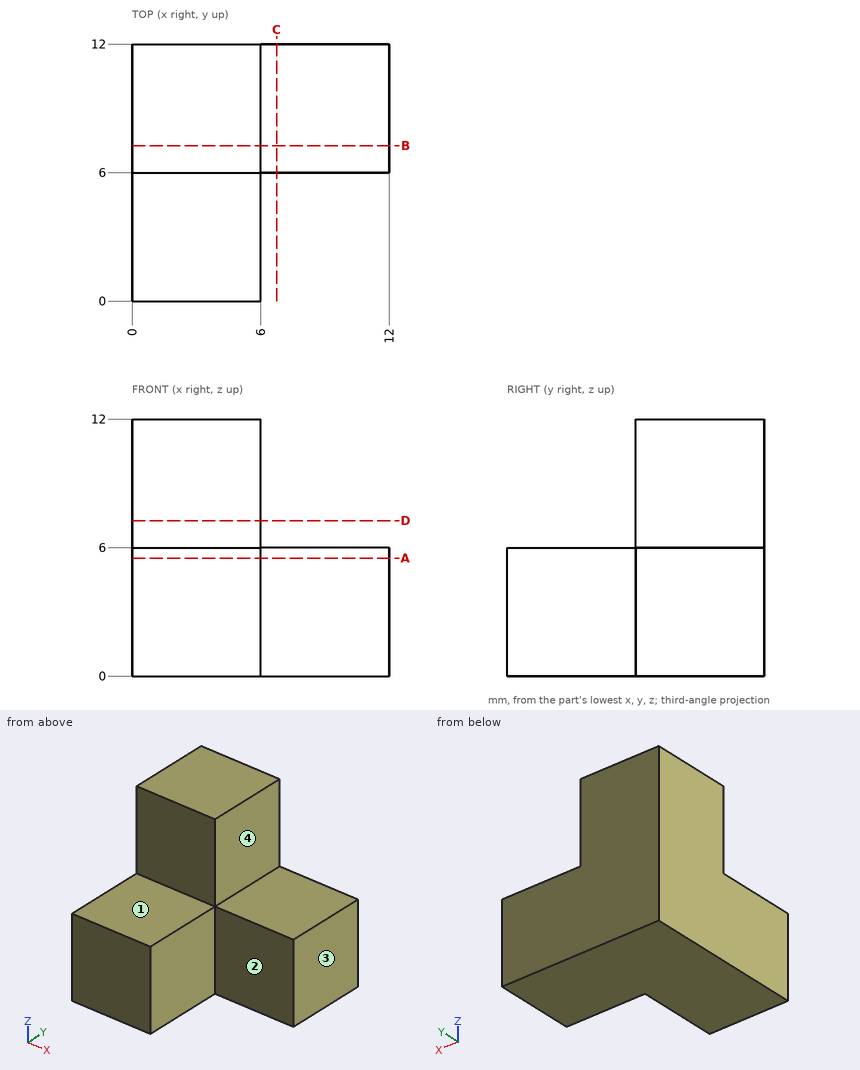
Study the drawing (mm; zero at the part's minimum x, y, z) and answer. A direction names the side the tool comes from. Coordinates: 2 decimals unless noted, no trailing zeros. Write each loop counter-clockwise with the first axis right and the second up, starting at its lowest first coordinate (ties: lowest second). Pieces come first, ordered by that corner, then holes. Notation, with made-up numbers: M -24.75,53 L 33.25,53 A36 ccw 33.25,89 Z; hole C 44.25,43 d10. An arc over 180 degrees is marked long. Use a Markdown table: item, result. Add a question column.
1. Section C-C (x = 6.75) is taken. Give the vertices of the cut face in (y, z), plus the area to 3 significant figures.
2. Section B-B (y = 7.25) is taken. Give the vertices of the cut face in (x, z), plus the area to 3 significant figures.
3. Section D-D (z = 7.25) is taken. Give the vertices of the cut face in (x, y).
4. Given P1, Ø3, axis at y = 4, z = 2, coming from the +X side; P2, Ø1.8, axis at x = 9.5, z = 3.5, coming from the -Y side; P3, Ø3, axis at x = 2.5, y = 3.5, coming from the +Z side, each flat-ended and moving along its own axis, determine where each tip first touches the part or whether it passes through.
5. Straight lines are drawn through the part: line 1 along Y through (x, z) = (2, 11); line 2 along X through (y, z) = (8.75, 11). For each, find the intervals that lie inside material, in ascending order. Write a range as [from, to].
6. Section A-A (z = 5.5) is taken. Give the vertices of the cut face in (x, y).
7. Which of the six approach directions +Z, -Z, +X, -X, +Y, -Y give full straight-line access (tool end or side, diameter ignored) to the marked faces 1, 2, 3 and 4?
Data:
| question | item | result |
|---|---|---|
| 1 | outline | M 6,0 L 12,0 L 12,6 L 6,6 Z |
| 1 | area | 36.0 mm2 |
| 2 | outline | M 0,0 L 12,0 L 12,6 L 6,6 L 6,12 L 0,12 Z |
| 2 | area | 108 mm2 |
| 3 | outline | M 0,6 L 6,6 L 6,12 L 0,12 Z |
| 4 | P1 | stops at x = 6 |
| 4 | P2 | stops at y = 6 |
| 4 | P3 | stops at z = 6 |
| 5 | line 1 | y = [6, 12] |
| 5 | line 2 | x = [0, 6] |
| 6 | outline | M 0,0 L 6,0 L 6,6 L 12,6 L 12,12 L 0,12 Z |
| 7 | face 1 | +Z, +X, -X, -Y |
| 7 | face 2 | +Z, -Z, +X, -Y |
| 7 | face 3 | +Z, -Z, +X, +Y, -Y |
| 7 | face 4 | +Z, +X, +Y, -Y |
